The listing builds one solid part. Answer for the finished solid, in the listing's coordinates (mm). Give positions to 0.01 mm unless a question says otherwise; leave off trailing zeros. Loops run counter-clockwise (first coordinate to the right, second up) from the corner with the lowest first, then second, coordinate; pieces in that order, holes last. Notation, with made-up numbers: (7, 62.25) - (23, 62.25) arc R32 cw to (23, 90.25) - close; hole circle Ø7 at (-25.75, -7). An arc over 180 degrees is marked (long way). Write each question's results on one line, items separated by ' | '.
from build123d import *

# Parameters (mm, degrees)
SKETCH1_R             = 97.5
BOSS_EXTRUDE1_DEPTH   = 8
SKETCH2_R             = 12.5
CUT_EXTRUDE1_DEPTH    = 139.117703427
SKETCH3_R             = 3.441916601
CUT_EXTRUDE2_DEPTH    = 5.339202
CIRPATTERN1_START     = 2.660798307
CIRPATTERN1_OUTLINE_R = 3.441916601
CIRPATTERN1_DEPTH     = 5.339201693


# Read off the part's stored shape, not the designer's step: CirPattern1
with BuildPart() as part:
    # Sketch1 → Boss-Extrude1 (new body)
    with BuildSketch(Plane(origin=(0, 0, 0), x_dir=(1, 0, 0), z_dir=(0, 1, 0))):
        with Locations(Location((0, 0, 0), (0, 0, 270))):
            Circle(SKETCH1_R)
    extrude(amount=BOSS_EXTRUDE1_DEPTH)

    # Sketch2 → Cut-Extrude1 (cut, through all)
    with BuildSketch(Plane(origin=(0, 0, 0), x_dir=(1, 0, 0), z_dir=(0, 1, 0))):
        with Locations(Location((0, 0, 0), (0, 0, 270))):
            Circle(SKETCH2_R)
    extrude(amount=CUT_EXTRUDE1_DEPTH, mode=Mode.SUBTRACT)

    # Sketch3 → Cut-Extrude2 (cut)
    with BuildSketch(Plane(origin=(0, 8, 0), x_dir=(1, 0, 0), z_dir=(0, 1, 0))):
        with Locations(Location((-26.305499443, 0, 0), (0, 0, 270))):
            Circle(SKETCH3_R)
    extrude(amount=-CUT_EXTRUDE2_DEPTH, mode=Mode.SUBTRACT)

    # CirPattern1 outline → CirPattern1 (cut)
    with BuildSketch(Plane(origin=(0, 0, 0), x_dir=(1, 0, 0), z_dir=(0, 1, 0)).offset(CIRPATTERN1_START)):
        with Locations((-18.600797039, -18.600797039)):
            Circle(CIRPATTERN1_OUTLINE_R)
        with Locations((-18.600797039, 18.600797039)):
            Circle(CIRPATTERN1_OUTLINE_R)
        with Locations((0, 26.305499443)):
            Circle(CIRPATTERN1_OUTLINE_R)
        with Locations((18.600797039, 18.600797039)):
            Circle(CIRPATTERN1_OUTLINE_R)
        with Locations((26.305499443, 0)):
            Circle(CIRPATTERN1_OUTLINE_R)
        with Locations((18.600797039, -18.600797039)):
            Circle(CIRPATTERN1_OUTLINE_R)
        with Locations((0, -26.305499443)):
            Circle(CIRPATTERN1_OUTLINE_R)
    extrude(amount=CIRPATTERN1_DEPTH, mode=Mode.SUBTRACT)


solid = part.part
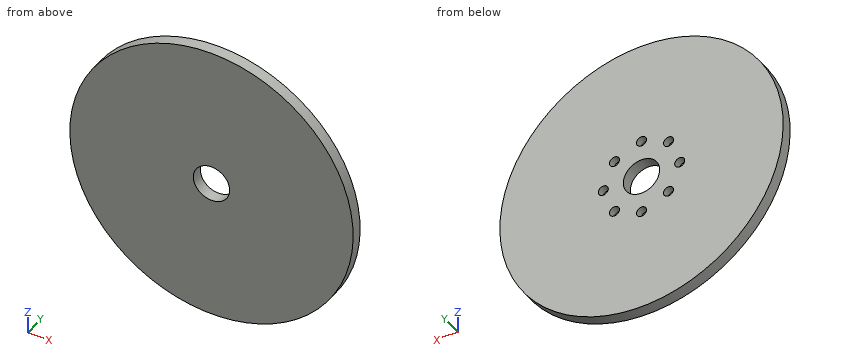
Item 1: A cutting plane is placed at C-C, the plane y = 6.5. Count the separate pieces of the cut face and the enclosed holes in it, plus the area to 3 significant figures.
Values found:
separate pieces: 1 | enclosed holes: 9 | area: 29,100 mm²
Item 2: Find the intervals of material crossed by line 1 along Z through (x, y) = (-18, 6.5); line 2 along Z through (x, y) = (10.5, 6.75); line 3 along X through (y, z) = (1.75, -2), in increasing order. Write a range as [from, to].
Values found:
line 1: z = [-95.82, -21.99], [-15.21, 15.21], [21.99, 95.82] | line 2: z = [-96.93, -6.78], [6.78, 96.93] | line 3: x = [-97.48, -12.34], [12.34, 97.48]
Item 3: A cutting plane is placed at A-A, the plane z = 0. Determine the outline of the cut face in (x, y), plus the area to 3 significant figures.
Values found:
outline: (-97.5, 0) - (-12.5, 0) - (-12.5, 8) - (-22.86, 8) - (-22.86, 2.66) - (-29.75, 2.66) - (-29.75, 8) - (-97.5, 8) - close; (12.5, 0) - (97.5, 0) - (97.5, 8) - (29.75, 8) - (29.75, 2.66) - (22.86, 2.66) - (22.86, 8) - (12.5, 8) - close | area: 1,290 mm²
Item 4: A cutting plane is placed at B-B, the plane x = 0. Determine the outline of the cut face in (y, z), plus the area to 3 significant figures.
Values found:
outline: (0, -97.5) - (8, -97.5) - (8, -29.75) - (2.66, -29.75) - (2.66, -22.86) - (8, -22.86) - (8, -12.5) - (0, -12.5) - close; (0, 12.5) - (8, 12.5) - (8, 22.86) - (2.66, 22.86) - (2.66, 29.75) - (8, 29.75) - (8, 97.5) - (0, 97.5) - close | area: 1,290 mm²
Item 5: Flat-ended cylindrical pins translate along their axes: P1, Ø4, axis at y = 3.5, z = 30.5, coming from the -X side; P2, Ø15, axis at x = 0, z = 0, coming from the +Y side; P3, Ø5.5, axis at x = -26.31, z = 0, coming from the +Y side. Find the tip coordinate at first contact, or state that the pin passes through.
Values found:
P1: stops at x = -93.24 | P2: passes through | P3: stops at y = 2.66
Item 6: A cutting plane is placed at D-D, the plane z = -67. Determine the outline of the cut face in (x, y), plus the area to 3 significant figures.
Values found:
outline: (-70.83, 0) - (70.83, 0) - (70.83, 8) - (-70.83, 8) - close | area: 1,130 mm²
